Read the model definition and answer for the solid it produces. Units are mm, in the model's axes. Face numbers are marked on the shaded views. Round coordinates to 2 decimals unless told otherwise and drop trailing zeros. Write each loop counter-clockwise with the first axis right and the second up, starting at its lowest first coordinate (ties: lowest second). Pieces come first, ordered by that corner, then holes. Notation, with made-up numbers: (29, -32) - (70, -32) arc R16 ccw to (70, -6) - close; hole circle Ø2 at (-10, 26.5). An arc over 180 degrees is marked (long way). Answer as CSV lines item,"result". Start each with the question number.
1) Find section C-C on x = -9.5. Determine the outline of the cut face in (y, z), then the cut area to 3 significant figures.
2) Each of these flat-tipped pins is pushed along its axis until it touches: pin 1 (3 mm diameter, centred on y = 9, z = 4.5, fed in from +X); pin 2 (1.5 mm diameter, centred on y = -6, z = 2.5, fed in from +X). Where does it stop, or does it pass through?
3) Find section D-D on y = 6. Determine the outline of the cut face in (x, z), then the cut area to 3 significant figures.
4) Find section B-B on z = 3.35. Determine the outline of the cut face in (x, y), then the cut area to 3 significant figures.
5) For a pull along X with two mould halves and no side action, classify the marked faces 1, 2 and 3 as +X half, -X half, draft (parallel to the pull), parting line (faces both ways), or undercut.
6) Consider line 1 along X through (y, z) = (-1.5, 1.05); line 2 along Y through (x, z) = (0, 3.6); line 3 along Y through (x, z) = (4, 1.25). Determine where each line is inside the solid, lowest interval first.
7) Find section A-A on y = -7.5. Determine the outline of the cut face in (x, z), then the cut area to 3 significant figures.
from build123d import *

# Parameters (mm, degrees)
SCHIZZO1_R                   = 2.05
ESTRUSIONE_ESTRUSIONE1_DEPTH = 5
CUT_EXTRUDE1_REACH           = 7
SKETCH1_R                    = 2.05


with BuildPart() as part:
    # Schizzo1 → Estrusione-Estrusione1 (new body)
    with BuildSketch(Plane.XY):
        with BuildLine():
            Line((0, -15), (49.434299833, -15))
            ThreePointArc((49.434299833, -15), (56.874189574, -6.552349937), (47.554189972, -0.239477504))
            ThreePointArc((47.554189972, -0.239477504), (27.787162994, 0.02445935), (10.90104019, 10.30375285))
            ThreePointArc((10.90104019, 10.30375285), (-13.775998925, 5.934800218), (0, -15))
        make_face()
        Circle(SCHIZZO1_R, mode=Mode.SUBTRACT)
        with Locations((49.434299833, -7.5)):
            Circle(SCHIZZO1_R, mode=Mode.SUBTRACT)
    extrude(amount=ESTRUSIONE_ESTRUSIONE1_DEPTH)

    # Sketch1 → Cut-Extrude1 (cut, up to next)
    with BuildSketch(Plane.XY.offset(5), mode=Mode.PRIVATE) as cut_extrude1_sk1:
        with Locations((4.608166562, -0.699135)):
            Circle(SKETCH1_R)
    cut_extrude1_tool1 = extrude(cut_extrude1_sk1.sketch, amount=-CUT_EXTRUDE1_REACH, mode=Mode.PRIVATE) & part.part
    add(cut_extrude1_tool1.solids().sort_by_distance((4.608167, -0.699135, 5))[0], mode=Mode.SUBTRACT)
    # Sketch1 → Cut-Extrude1 (cut, up to next)
    with BuildSketch(Plane.XY.offset(5), mode=Mode.PRIVATE) as cut_extrude1_sk2:
        with Locations((12.141953856, -1.842135)):
            Circle(SKETCH1_R)
    cut_extrude1_tool2 = extrude(cut_extrude1_sk2.sketch, amount=-CUT_EXTRUDE1_REACH, mode=Mode.PRIVATE) & part.part
    add(cut_extrude1_tool2.solids().sort_by_distance((12.141954, -1.842135, 5))[0], mode=Mode.SUBTRACT)


solid = part.part
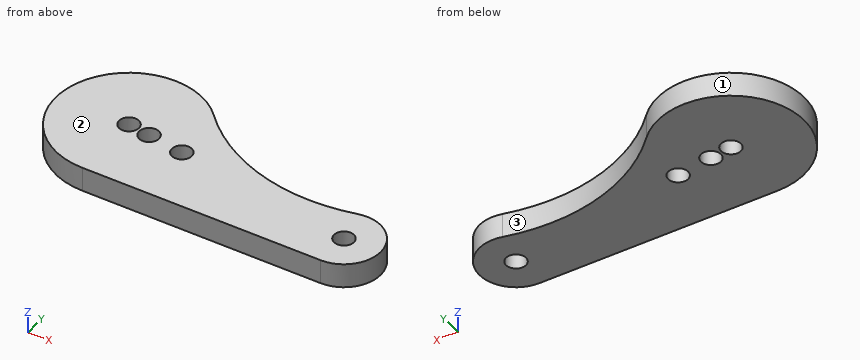
Check values:
1,outline,"(-11.61, 0) - (11.61, 0) - (11.61, 5) - (-11.61, 5) - close"
1,area,"116 mm^2"
2,pin 1,"stops at x = 13.86"
2,pin 2,"stops at x = 56.9"
3,outline,"(-13.75, 0) - (15.74, 0) - (15.74, 5) - (-13.75, 5) - close"
3,area,"147 mm^2"
4,outline,"(0, -15) - (49.43, -15) arc R7.5 ccw (long way) to (47.55, -0.24) arc R37.5 cw to (10.9, 10.3) arc R15 ccw (long way) to start; hole circle Ø4.1 at (0, 0); hole circle Ø4.1 at (4.61, -0.7); hole circle Ø4.1 at (12.14, -1.84); hole circle Ø4.1 at (49.43, -7.5)"
4,area,"1,330 mm^2"
5,face 1,"parting line"
5,face 2,"draft"
5,face 3,"undercut"
6,line 1,"x = -14.92 to -1.4, 1.4 to 2.72, 6.5 to 10.12, 14.16 to 53.93"
6,line 2,"y = -15 to -2.05, 2.05 to 15"
6,line 3,"y = -15 to -2.66, 1.26 to 14.46"
7,outline,"(-12.99, 0) - (47.38, 0) - (47.38, 5) - (-12.99, 5) - close; (51.48, 0) - (56.93, 0) - (56.93, 5) - (51.48, 5) - close"
7,area,"329 mm^2"
